from build123d import *

# Parameters (mm, degrees)
F0_W        = 20.9599784
F0_H        = 42.260012
F0_R        = 2.032
F1_DEPTH    = 6.35
F2_W        = 32.0040006191
F2_H        = 57.15
F2_W_2      = 20.9599784
F2_H_2      = 42.260012
F3_DEPTH    = 12.7
F4_W        = 54.2940877291
F4_H        = 95.895376205
F4_W_2      = 32.0040006191
F4_H_2      = 57.15
F4_R        = 2.032
F3_FACE_W   = 32.0040006191
F3_FACE_H   = 57.15
F3_FACE_W_2 = 20.9599784
F3_FACE_H_2 = 42.260012
F5_DEPTH    = 25.4


with BuildPart() as f1:
    # F0 (on Top) → F1 (new body)
    with BuildSketch(Plane.XY):
        Polygon((64.1610962078, 69.1004172512), (36.6851288078, 69.1004172512), (9.8670084787, 69.1004172512), (9.8670084787, 61.6404372512), (9.8670084787, -26.7949589538), (64.1610962078, -26.7949589538), align=None)
        with Locations((47.1651180078, 4.2184540512)):
            Rectangle(F0_W, F0_H, mode=Mode.SUBTRACT)
        with BuildLine():
            ThreePointArc((34.2246816078, 61.6404372512), (32.1926816078, 59.6084372512), (30.1606816078, 61.6404372512))
            ThreePointArc((30.1606816078, 61.6404372512), (32.1926816078, 63.6724372512), (34.2246816078, 61.6404372512))
        make_face(mode=Mode.SUBTRACT)
        with BuildLine():
            Line((9.8670084787, 61.6404372512), (9.8670084787, 69.1004172512))
            Line((9.8670084787, 69.1004172512), (-44.4270792504, 69.1004172512))
            Line((-44.4270792504, 69.1004172512), (-44.4270792504, -26.7949589538))
            Line((-44.4270792504, -26.7949589538), (-18.7219286708, -26.7949589538))
            Line((-18.7219286708, -26.7949589538), (-18.7219286708, 59.6084372512))
            ThreePointArc((-18.7219286708, 59.6084372512), (-20.1587696502, 63.0772782306), (-16.6899286708, 61.6404372512))
            Line((-16.6899286708, 61.6404372512), (9.8670084787, 61.6404372512))
        make_face()
        with Locations((-34.6146070708, -4.524490289)):
            Circle(F0_R, mode=Mode.SUBTRACT)
        with BuildLine():
            Line((9.8670084787, -26.7949589538), (9.8670084787, 61.6404372512))
            Line((9.8670084787, 61.6404372512), (-16.6899286708, 61.6404372512))
            ThreePointArc((-16.6899286708, 61.6404372512), (-17.2850876915, 60.2035962718), (-18.7219286708, 59.6084372512))
            Line((-18.7219286708, 59.6084372512), (-18.7219286708, -26.7949589538))
            Line((-18.7219286708, -26.7949589538), (9.8670084787, -26.7949589538))
        make_face()
    extrude(amount=F1_DEPTH)

    # F2 (on face) → F3 (join)
    with BuildSketch(Plane.XY.offset(6.35)):
        with Locations((47.0991291173, 4.2974480512)):
            Rectangle(F2_W, F2_H)
        with Locations((47.1651180078, 4.2184540512)):
            Rectangle(F2_W_2, F2_H_2, mode=Mode.SUBTRACT)
    extrude(amount=F3_DEPTH)

    # F4 (on face) + F3_face (on face) → F5 (cut)
    with BuildSketch(Plane.XY.offset(6.35)):
        with Locations((37.0140523432, 21.1527291487)):
            Rectangle(F4_W, F4_H)
        with Locations((47.0991291173, 4.2974480512)):
            Rectangle(F4_W_2, F4_H_2, mode=Mode.SUBTRACT)
        with Locations((32.1926816078, 61.6404372512)):
            Circle(F4_R, mode=Mode.SUBTRACT)
    with BuildSketch(Plane(origin=(47.0371621853, 4.371627444, 19.05), x_dir=(1, 0, 0), z_dir=(0, 0, 1))):
        with Locations((0.061966932, -0.0741793928)):
            Rectangle(F3_FACE_W, F3_FACE_H)
        with Locations((0.1279558225, -0.1531733928)):
            Rectangle(F3_FACE_W_2, F3_FACE_H_2, mode=Mode.SUBTRACT)
    extrude(amount=-F5_DEPTH, mode=Mode.SUBTRACT)


solid = f1.part
Geometry check sheet. Reference: the model listing, model coordinates, mm. Give positions to 0.01 mm unless a question says otherwise; leave off trailing zeros. Write each loop counter-clockwise with the first axis right and the second up, starting at its lowest first coordinate (ties: lowest second). Pieces come first, ordered by that corner, then holes.
1) Thickness scan on line 1 (Y direction, x = -20.5, z = 3.75); line 2 (Y direction, x = -18, z = 5.5); line 3 (X direction, y = 61, z = 5.25). Record the ranges inside material, lowest first.
Values follow:
line 1: y = -26.79 to 60.66, 62.62 to 69.1
line 2: y = -26.79 to 59.74, 63.54 to 69.1
line 3: x = -44.43 to -20.65, -16.79 to 9.87
2) Cross-section at A-A (y = -5.5). Record the boundary of the cut face in (x, z), plus the area to 3 significant figures.
Values follow:
outline: (-44.43, 0) - (-36.4, 0) - (-36.4, 6.35) - (-44.43, 6.35) - close; (-32.83, 0) - (9.87, 0) - (9.87, 6.35) - (-32.83, 6.35) - close
area: 322 mm2
3) Release check for a two-part mould opening along X. For faces 1 (the face through (-18, 22, 0)), 2 (the face through (-36.645, -4.435, 3.131)), 3 (the face through (9.867, 20, 3)) record: released by +X, released by -X, zero draft, split by the parting line, or undercut.
Values follow:
face 1: zero draft
face 2: undercut
face 3: released by +X
